```python
from build123d import *

# Parameters (mm, degrees)
F0_W     = 59
F0_H     = 69
F0_R     = 1
F1_DEPTH = 1.5
F2_W     = 8
F2_H     = 1.5
F2_H_2   = 4.5
F3_DEPTH = 3
F2_W_2   = 15.5
F2_H_3   = 16.5
F2_H_4   = 0.5
F4_DEPTH = 16.5
F2_W_3   = 16
F2_H_5   = 19.5
F5_DEPTH = 13
F2_W_4   = 0.5
F2_H_6   = 26
F2_W_5   = 8.5
F6_DEPTH = 2.5


with BuildPart() as f1:
    # F0 (on Top) → F1 (new body)
    with BuildSketch(Plane.XY):
        Rectangle(F0_W, F0_H)
        with Locations((-26.5, -31.5)):
            Circle(F0_R, mode=Mode.SUBTRACT)
        with Locations((26.5, -31.5)):
            Circle(F0_R, mode=Mode.SUBTRACT)
        with Locations((-13.5, 21.5)):
            Circle(F0_R, mode=Mode.SUBTRACT)
        with Locations((26.5, 31.5)):
            Circle(F0_R, mode=Mode.SUBTRACT)
    extrude(amount=F1_DEPTH)

    # F2 (on face) → F3 (join)
    with BuildSketch(Plane.XY.offset(1.5)):
        with Locations((19.5, -35.25)):
            Rectangle(F2_W, F2_H)
        with Locations((19.5, -32.25)):
            Rectangle(F2_W, F2_H_2)
    extrude(amount=F3_DEPTH)

    # F2 (on face) → F4 (join)
    with BuildSketch(Plane.XY.offset(1.5)):
        with Locations((4.75, -26.25)):
            Rectangle(F2_W_2, F2_H_3)
        with Locations((4.75, -34.75)):
            Rectangle(F2_W_2, F2_H_4)
    extrude(amount=F4_DEPTH)

    # F2 (on face) → F5 (join)
    with BuildSketch(Plane.XY.offset(1.5)):
        with Locations((-15.5, -24.75)):
            Rectangle(F2_W_3, F2_H_5)
        with Locations((-15.5, -35.25)):
            Rectangle(F2_W_3, F2_H)
    extrude(amount=F5_DEPTH)

    # F2 (on face) → F6 (join)
    with BuildSketch(Plane.XY.offset(1.5)):
        with Locations((29.25, 15.5)):
            Rectangle(F2_W_4, F2_H_6)
        with Locations((33.75, 15.5)):
            Rectangle(F2_W_5, F2_H_6)
        with Locations((29.25, -15.5)):
            Rectangle(F2_W_4, F2_H_6)
        with Locations((33.75, -15.5)):
            Rectangle(F2_W_5, F2_H_6)
    extrude(amount=F6_DEPTH)


solid = f1.part
```
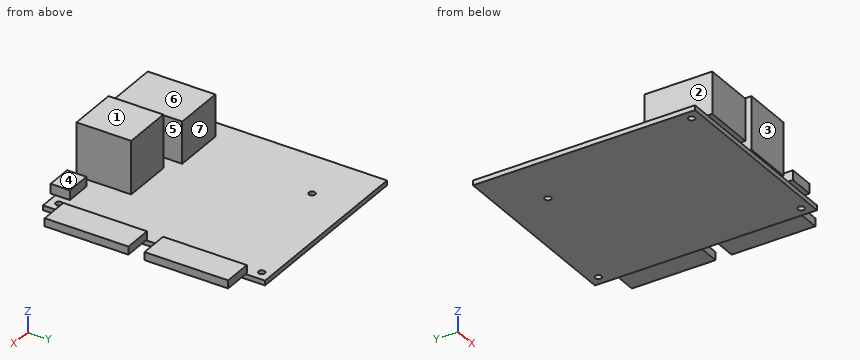
Source: CAD feature listing. Evaluate the final solid. Frame: model axes, mm. Face numbers are marked on the shaded views. A direction names the side the tool comes from. Round coordinates to 2 decimals unless told otherwise and drop trailing zeros. Loops run counter-clockwise (first coordinate to the right, second up) from the corner with the lowest first, then second, coordinate; pieces in that order, holes last.
1. Ray query, L1, parallel to Y at x = 26.5, z = 0.35; L2, parallel to X at y = -25.5, z = 11.25; L3, parallel to Y at x = -26.5, z = 0.85. Return the intervals inside material, ascending.
2. Section query A-A on y = -31.5. Output: boundary loops of the cut face in (x, z), and give its area (3 significant figures).
3. Section query B-B on x = 26.5. Output: boundary loops of the cut face in (y, z).
4. Section query C-C on y = 21.5. Output: boundary loops of the cut face in (x, z).
5. Access query for the marked faces 4, 5, 6 and 7. Directions: +Z, -Z, +X, -X, +Y, -Y. A direction counts if a zero-diameter tool reaches every point of the face in a straight line with its end or side. Return the directions, or none.
6. Contact query for flat-ended pins moving along their axis: pin 1 (5 mm diameter, centred on x = -13.5, y = 14.5, fed in from +Z); pin 2 (1.6 mm diameter, centred on x = 6, z = 0.5, fed in from -Y); pin 3 (5 mm diameter, centred on x = -12.5, y = -29.5, fed in from +Z); pin 4 (1.6 mm diameter, centred on x = -13.5, y = 21.5, fed in from -Z). Output: stop coordinate, or through.
7. Section query D-D on z = 6.25. Output: boundary loops of the cut face in (x, y), and give its area (4 significant figures).
8. Mould query, pull axis X, two halves, no side actions, for the marked faces 1, 2 and 3. Classes: released by +X, released by -X, zero draft, split by the parting line, or undercut.
Answers below:
1. L1: y = -34.5 to -32.5, -30.5 to 30.5, 32.5 to 34.5
1. L2: x = -23.5 to -7.5, -3 to 12.5
1. L3: y = -34.5 to -32.5, -30.5 to 34.5
2. outline: (-29.5, 0) - (-27.5, 0) - (-27.5, 1.5) - (-29.5, 1.5) - close; (-25.5, 0) - (25.5, 0) - (25.5, 1.5) - (23.5, 1.5) - (23.5, 4.5) - (15.5, 4.5) - (15.5, 1.5) - (12.5, 1.5) - (12.5, 18) - (-3, 18) - (-3, 1.5) - (-7.5, 1.5) - (-7.5, 14.5) - (-23.5, 14.5) - (-23.5, 1.5) - (-25.5, 1.5) - close; (27.5, 0) - (29.5, 0) - (29.5, 1.5) - (27.5, 1.5) - close
2. area: 570 mm2
3. outline: (-34.5, 0) - (-32.5, 0) - (-32.5, 1.5) - (-34.5, 1.5) - close; (-30.5, 0) - (30.5, 0) - (30.5, 1.5) - (-30.5, 1.5) - close; (32.5, 0) - (34.5, 0) - (34.5, 1.5) - (32.5, 1.5) - close
4. outline: (-29.5, 0) - (-14.5, 0) - (-14.5, 1.5) - (-29.5, 1.5) - close; (-12.5, 0) - (29.5, 0) - (29.5, 1.5) - (38, 1.5) - (38, 4) - (29, 4) - (29, 1.5) - (-12.5, 1.5) - close
5. face 4: +Z, +X, +Y, -Y
5. face 5: +Z, +Y, -Y
5. face 6: +Z, -X, +Y, -Y
5. face 7: +Z, -X, +Y
6. pin 1: stops at z = 1.5
6. pin 2: stops at y = -34.5
6. pin 3: stops at z = 14.5
6. pin 4: passes through
7. outline: (-23.5, -36) - (-7.5, -36) - (-7.5, -15) - (-23.5, -15) - close; (-3, -35) - (12.5, -35) - (12.5, -18) - (-3, -18) - close
7. area: 599.5 mm2
8. face 1: zero draft
8. face 2: released by -X
8. face 3: undercut
